from build123d import *

# Parameters (mm, degrees)
SKETCH2_R           = 75
SKETCH2_R_2         = 3.5687
SKETCH2_R_3         = 4.8
BOSS_EXTRUDE1_DEPTH = 4.7625
SKETCH3_R           = 1.5
CUT_EXTRUDE1_DEPTH  = 107.172884515
SKETCH4_R           = 1.7
CUT_EXTRUDE2_DEPTH  = 107.172884515
SKETCH5_R           = 1.7
CUT_EXTRUDE3_DEPTH  = 107.172884515
SKETCH6_R           = 1.75
CUT_EXTRUDE4_DEPTH  = 107.172884515
SKETCH7_R           = 3.25
SKETCH7_R_2         = 1.7272
BOSS_EXTRUDE2_DEPTH = 10
CUT_EXTRUDE5_DEPTH  = 10


# Read off the part's stored shape, not the designer's step: Draft1
with BuildPart() as part:
    # Sketch2 → Boss-Extrude1 (new body)
    with BuildSketch(Plane.XY.offset(157.1625)):
        with Locations(Location((0, 0, 0), (0, 0, 180))):
            Circle(SKETCH2_R)
        with Locations(Location((0, 50, 0), (0, 0, 180))):
            Circle(SKETCH2_R_2, mode=Mode.SUBTRACT)
        with Locations(Location((0, -50, 0), (0, 0, 180))):
            Circle(SKETCH2_R_2, mode=Mode.SUBTRACT)
        with Locations(Location((25.102290732, 25.102290732, 0), (0, 0, 180))):
            Circle(SKETCH2_R_3, mode=Mode.SUBTRACT)
        with Locations(Location((-25.102290732, 25.102290732, 0), (0, 0, 180))):
            Circle(SKETCH2_R_3, mode=Mode.SUBTRACT)
        with Locations(Location((-25.102290732, -25.102290732, 0), (0, 0, 180))):
            Circle(SKETCH2_R_3, mode=Mode.SUBTRACT)
        with Locations(Location((25.102290732, -25.102290732, 0), (0, 0, 180))):
            Circle(SKETCH2_R_3, mode=Mode.SUBTRACT)
    extrude(amount=BOSS_EXTRUDE1_DEPTH)

    # Sketch3 → Cut-Extrude1 (cut, through all)
    with BuildSketch(Plane.XY.offset(161.925)):
        with Locations((14.849242405, 14.849242405)):
            Circle(SKETCH3_R)
        with Locations((-14.849242405, 14.849242405)):
            Circle(SKETCH3_R)
        with Locations((-14.849242405, -14.849242405)):
            Circle(SKETCH3_R)
        with Locations((14.849242405, -14.849242405)):
            Circle(SKETCH3_R)
    extrude(amount=-CUT_EXTRUDE1_DEPTH, mode=Mode.SUBTRACT)

    # Sketch4 → Cut-Extrude2 (cut, through all)
    with BuildSketch(Plane.XY.offset(161.925)):
        with Locations((0, 25)):
            Circle(SKETCH4_R)
        with Locations((25, 0)):
            Circle(SKETCH4_R)
        with Locations((0, -25)):
            Circle(SKETCH4_R)
        with Locations((-25, 0)):
            Circle(SKETCH4_R)
    extrude(amount=-CUT_EXTRUDE2_DEPTH, mode=Mode.SUBTRACT)

    # Sketch5 → Cut-Extrude3 (cut, through all)
    with BuildSketch(Plane.XY.offset(161.925)):
        with Locations((-35, 0)):
            Circle(SKETCH5_R)
        with Locations((-55, 0)):
            Circle(SKETCH5_R)
        with Locations((35, 0)):
            Circle(SKETCH5_R)
        with Locations((55, 0)):
            Circle(SKETCH5_R)
    extrude(amount=-CUT_EXTRUDE3_DEPTH, mode=Mode.SUBTRACT)

    # Sketch6 → Cut-Extrude4 (cut, through all)
    with BuildSketch(Plane.XY.offset(161.925)):
        with Locations((0, 68.825)):
            Circle(SKETCH6_R)
        with Locations((68.825, 0)):
            Circle(SKETCH6_R)
        with Locations((0, -68.825)):
            Circle(SKETCH6_R)
        with Locations((-68.825, 0)):
            Circle(SKETCH6_R)
    extrude(amount=-CUT_EXTRUDE4_DEPTH, mode=Mode.SUBTRACT)

    # Sketch7 → Boss-Extrude2 (add)
    # profile 1 of 4: a face of its own
    with BuildSketch(Plane(origin=(0, 0, 157.1625), x_dir=(-1, 0, 0), z_dir=(0, 0, -1))):
        with Locations(Location((7.424621202, -7.424621202, 0), (0, 0, 180))):
            Circle(SKETCH7_R)
        with Locations((7.424621202, -7.424621202)):
            Circle(SKETCH7_R_2, mode=Mode.SUBTRACT)
    # profile 2 of 4: a face of its own
    with BuildSketch(Plane(origin=(0, 0, 157.1625), x_dir=(-1, 0, 0), z_dir=(0, 0, -1))):
        with Locations(Location((7.424621202, 7.424621202, 0), (0, 0, 180))):
            Circle(SKETCH7_R)
        with Locations((7.424621202, 7.424621202)):
            Circle(SKETCH7_R_2, mode=Mode.SUBTRACT)
    # profile 3 of 4: a face of its own
    with BuildSketch(Plane(origin=(0, 0, 157.1625), x_dir=(-1, 0, 0), z_dir=(0, 0, -1))):
        with Locations(Location((-7.424621202, 7.424621202, 0), (0, 0, 180))):
            Circle(SKETCH7_R)
        with Locations((-7.424621202, 7.424621202)):
            Circle(SKETCH7_R_2, mode=Mode.SUBTRACT)
    # profile 4 of 4: a face of its own
    with BuildSketch(Plane(origin=(0, 0, 157.1625), x_dir=(-1, 0, 0), z_dir=(0, 0, -1))):
        with Locations(Location((-7.424621202, -7.424621202, 0), (0, 0, 180))):
            Circle(SKETCH7_R)
        with Locations((-7.424621202, -7.424621202)):
            Circle(SKETCH7_R_2, mode=Mode.SUBTRACT)
    extrude(amount=BOSS_EXTRUDE2_DEPTH)

    # Sketch8 → Cut-Extrude5 (cut)
    with BuildSketch(Plane(origin=(0, 0, 157.1625), x_dir=(-1, 0, 0), z_dir=(0, 0, -1))):
        Polygon((-12.765502036, 56.949907443), (-31.243092686, 49.296238796), (-33.156509848, 53.915636458), (-14.678919198, 61.569305106), align=None)
    extrude(amount=-CUT_EXTRUDE5_DEPTH, mode=Mode.SUBTRACT)

    # Draft1 outline → Draft1 (revolve)
    with BuildSketch(Plane(origin=(-7.424621202, -7.424621202, 0), x_dir=(1, 0, 0), z_dir=(0, -1, 0))):
        Polygon((3.25, 157.1625), (3.25, 147.1625), (5.929491924, 157.1625), align=None)
    revolve(axis=Axis((-7.424621202, -7.424621202, 0), (0, 0, 1)))

    # Draft1 2 outline → Draft1 2 (revolve)
    with BuildSketch(Plane(origin=(-7.424621202, 7.424621202, 0), x_dir=(1, 0, 0), z_dir=(0, -1, 0))):
        Polygon((3.25, 157.1625), (3.25, 147.1625), (5.929491924, 157.1625), align=None)
    revolve(axis=Axis((-7.424621202, 7.424621202, 0), (0, 0, 1)))

    # Draft1 3 outline → Draft1 3 (revolve)
    with BuildSketch(Plane(origin=(7.424621202, 7.424621202, 0), x_dir=(1, 0, 0), z_dir=(0, -1, 0))):
        Polygon((3.25, 157.1625), (3.25, 147.1625), (5.929491924, 157.1625), align=None)
    revolve(axis=Axis((7.424621202, 7.424621202, 0), (0, 0, 1)))

    # Draft1 4 outline → Draft1 4 (revolve)
    with BuildSketch(Plane(origin=(7.424621202, -7.424621202, 0), x_dir=(1, 0, 0), z_dir=(0, -1, 0))):
        Polygon((3.25, 157.1625), (3.25, 147.1625), (5.929491924, 157.1625), align=None)
    revolve(axis=Axis((7.424621202, -7.424621202, 0), (0, 0, 1)))


solid = part.part
Check sheet for the modelled part. Datum: model origin and axes. Units: mm. A direction names the side the tool comes from. Coordinates: 2 decimals unless noted, no trailing zeros. Loops run counter-clockwise (first coordinate to the right, second up) from the corner with the lowest first, then second, coordinate; pieces in that order, holes last. Notation, with made-up numbers: (46, 49) -> (59, 49) arc R7 cw to (59, 58) -> close; hole circle Ø2 at (3, 41). An arc over 180 degrees is marked (long way). Write item = value, one per line. Start each with the question number.
1. Depth check by flat-ended pin: P1, Ø5.5, axis at x = 0, y = 25, coming from the +Z side (3 decimals); P2, Ø3, axis at x = 0, y = -25, coming from the -Z side; P3, Ø10, axis at x = -13.5, y = 46.5, coming from the -Z side; P4, Ø3, axis at y = 19, z = 158.5, coming from the -X side. Enter the tip coordinate at first touch or a pass-through.
2. Section check C-C on y = 36.5. Record the cut outline in (x, z) (1 decimal).
3. Material ranges on line 1 (X direction, y = -15.5, z = 157.25); line 2 (X direction, y = -22, z = 157.25); line 3 (Z direction, x = 52, y = -4) (1 decimal), recorded low to high.
4. Section check B-B on y = -32.5. Record the cut outline in (x, z) (1 decimal), then the cut area to 3 significant figures.
5. Tool access check on faces 4 (the flat face through (1, -1, 161.925)), 5 (the flat face through (24.047, 57.689, 159.51)), 6 (the cylindrical face through (-8.22, 5.89, 152.23)). Record the directions out of +Z, -Z, +X, -X, +Y, -Y that give a thin tool (end or side, any length) a straight path to the whole face; none if there is none.
6. Draft check along Y on faces 1 (the cylindrical face through (6.63, 5.89, 152.23)), 2 (the flat face through (9, 9, 147.162)), 3 (the flat face through (21.87, 53.18, 159.51)). Enter one of: released by +Y, released by -Y, zero draft, split by the parting line, or undercut.
7. Section check A-A on z = 153.75. Record the cut outline in (x, y).
Responses:
q1.P1 = 161.925
q1.P2 = through
q1.P3 = 157.16
q1.P4 = -72.93
q2.outline = (-65.5, 157.2) -> (65.5, 157.2) -> (65.5, 161.9) -> (-65.5, 161.9) -> close
q3.line_1 = -73.38 to -16.2, -13.5 to 13.5, 16.2 to 73.38
q3.line_2 = -71.7 to -28.77, -21.44 to 21.44, 28.77 to 71.7
q3.line_3 = 157.2 to 161.9
q4.outline = (-67.6, 157.2) -> (67.6, 157.2) -> (67.6, 161.9) -> (-67.6, 161.9) -> close
q4.area = 644 mm2
q5.face_4 = +Z, +X, -X, +Y, -Y
q5.face_5 = +Z, -Z
q5.face_6 = -Z
q6.face_1 = undercut
q6.face_2 = zero draft
q6.face_3 = undercut
q7.outline = circle Ø10.03 at (-7.42, -7.42); circle Ø10.03 at (-7.42, 7.42); circle Ø10.03 at (7.42, -7.42); circle Ø10.03 at (7.42, 7.42); hole circle Ø3.45 at (-7.42, -7.42); hole circle Ø3.45 at (-7.42, 7.42); hole circle Ø3.45 at (7.42, -7.42); hole circle Ø3.45 at (7.42, 7.42)
